from build123d import *

# Parameters (mm, degrees)
SKIZZE1_R                             = 44
AUFSATZ_LINEAR_AUSTRAGEN1_DEPTH       = 4
SCHNITT_LINEAR_START                  = -10
SCHNITT_LINEAR_AUSTRAGEN2_DEPTH       = 10
KREISMUSTER1_COUNT                    = 6
SCHNITT_LINEAR_AUSTRAGEN3_DEPTH       = 4
SCHNITT_LINEAR_AUSTRAGEN3_DEPTH_BACK  = 10
VERRUNDUNG1_R                         = 2
SKIZZE7_R                             = 32
SCHNITT_LINEAR_AUSTRAGEN7_DEPTH       = 0.5
SKIZZE8_R                             = 45
SKIZZE8_R_2                           = 43
AUFSATZ_LINEAR_AUSTRAGEN2_DEPTH       = 6
AUFSATZ_LINEAR_AUSTRAGEN3_DEPTH       = 9
AUFSATZ_LINEAR_AUSTRAGEN3_DEPTH_BACK  = 1
SKIZZE9_R                             = 45
SKIZZE9_R_2                           = 39.5
SKIZZE4_R                             = 21.007106764
AUFSATZ_LINEAR_AUSTRAGEN8_DEPTH       = 6
FASE1_SIZE                            = 3.25
SKIZZE10_R                            = 50
SKIZZE10_R_2                          = 42
SCHNITT_LINEAR_AUSTRAGEN9_DEPTH       = 8
SKIZZE11_R                            = 50
SKIZZE11_R_2                          = 40.9
SCHNITT_LINEAR_AUSTRAGEN10_DEPTH      = 2
SCHNITT_LINEAR_AUSTRAGEN11_DEPTH      = 6
SCHNITT_LINEAR_AUSTRAGEN11_DEPTH_BACK = 6
FASE3_SIZE                            = 2
FASE5_SIZE                            = 2
SKIZZE12_R                            = 2.5
SCHNITT_LINEAR_AUSTRAGEN12_DEPTH      = 79.994520679
VERRUNDUNG2_R                         = 1


with BuildPart() as part:
    # Skizze1 → Aufsatz-Linear austragen1 (new body)
    with BuildSketch(Plane(origin=(0, 0, 0), x_dir=(1, 0, 0), z_dir=(0, 1, 0))):
        with Locations(Location((0, 0, 0), (0, 0, 270))):
            Circle(SKIZZE1_R)
    extrude(amount=AUFSATZ_LINEAR_AUSTRAGEN1_DEPTH)

    # Skizze2 → Schnitt-Linear austragen2 (cut)
    with BuildSketch(Plane(origin=(0, 4, 0), x_dir=(1, 0, 0), z_dir=(0, 1, 0)).offset(SCHNITT_LINEAR_START)):
        with BuildLine():
            ThreePointArc((-30, 0), (-30.647234858, 7.855929826), (-32.571484726, 15.5))
            Line((-32.571484726, 15.5), (-41.179485184, 15.5))
            ThreePointArc((-41.179485184, 15.5), (-44, 0), (-41.179485184, -15.5))
            Line((-41.179485184, -15.5), (-32.571484726, -15.5))
            ThreePointArc((-32.571484726, -15.5), (-30.647234858, -7.855929826), (-30, 0))
        make_face()
    schnitt_linear_austragen2 = extrude(amount=SCHNITT_LINEAR_AUSTRAGEN2_DEPTH, mode=Mode.SUBTRACT)

    # Kreismuster1: Schnitt-Linear austragen2 ×6 about axis
    kreismuster1_axis = Axis((0, 0, 0), (0, 1, 0))
    for i in range(1, KREISMUSTER1_COUNT):
        add(schnitt_linear_austragen2.rotate(kreismuster1_axis, i * 360 / KREISMUSTER1_COUNT), mode=Mode.SUBTRACT)

    # Skizze3 → Schnitt-Linear austragen3 (cut, two sides: drawn at the far end of the back side and taken through both)
    with BuildSketch(Plane.XZ.offset(-SCHNITT_LINEAR_AUSTRAGEN3_DEPTH_BACK)):
        Polygon((15, 8.660254038), (0, 17.320508076), (-15, 8.660254038), (-15, -8.660254038), (0, -17.320508076), (15, -8.660254038), align=None)
    extrude(amount=SCHNITT_LINEAR_AUSTRAGEN3_DEPTH + SCHNITT_LINEAR_AUSTRAGEN3_DEPTH_BACK, mode=Mode.SUBTRACT)

    # Verrundung1
    verrundung1_edges = [part.edges().sort_by_distance(p)[0] for p in [
        (-32.571484726, 2, 15.5),
        (-32.571484726, 2, -15.5),
        (-29.709136122, 2, -20.457733212),
        (-2.862348604, 2, -35.957733212),
        (2.862348604, 2, -35.957733212),
        (29.709136122, 2, -20.457733212),
        (32.571484726, 2, -15.5),
        (32.571484726, 2, 15.5),
        (29.709136122, 2, 20.457733212),
        (2.862348604, 2, 35.957733212),
        (-2.862348604, 2, 35.957733212),
        (-29.709136122, 2, 20.457733212),
    ]]
    fillet(verrundung1_edges, radius=VERRUNDUNG1_R)

    # Skizze7 → Schnitt-Linear austragen7 (cut)
    with BuildSketch(Plane.XZ):
        Circle(SKIZZE7_R)
    extrude(amount=-SCHNITT_LINEAR_AUSTRAGEN7_DEPTH, mode=Mode.SUBTRACT)

    # Skizze8 → Aufsatz-Linear austragen2 (add)
    with BuildSketch(Plane(origin=(0, 4, 0), x_dir=(1, 0, 0), z_dir=(0, 1, 0))):
        with Locations(Location((0, 0, 0), (0, 0, 270))):
            Circle(SKIZZE8_R)
        with Locations(Location((0, 0, 0), (0, 0, 270))):
            Circle(SKIZZE8_R_2, mode=Mode.SUBTRACT)
    extrude(amount=-AUFSATZ_LINEAR_AUSTRAGEN2_DEPTH)



with BuildPart() as body_2:
    # Skizze9 → Aufsatz-Linear austragen3 (new, two sides: drawn at the far end of the back side and taken through both)
    with BuildSketch(Plane.XZ.offset(2).offset(-AUFSATZ_LINEAR_AUSTRAGEN3_DEPTH_BACK)):
        with Locations(Location((0, 0, 0), (0, 0, 90))):
            Circle(SKIZZE9_R)
        with Locations(Location((0, 0, 0), (0, 0, 270))):
            Circle(SKIZZE9_R_2, mode=Mode.SUBTRACT)
    extrude(amount=AUFSATZ_LINEAR_AUSTRAGEN3_DEPTH + AUFSATZ_LINEAR_AUSTRAGEN3_DEPTH_BACK)


with BuildPart() as part_1:
    add(part.part)

    add(body_2.part)  # Aufsatz-Linear austragen8 merges body 2
    # Skizze4 → Aufsatz-Linear austragen8 (add)
    with BuildSketch(Plane(origin=(0, 4, 0), x_dir=(1, 0, 0), z_dir=(0, 1, 0))):
        with Locations(Location((0, 0, 0), (0, 0, 270))):
            Circle(SKIZZE4_R)
    extrude(amount=-AUFSATZ_LINEAR_AUSTRAGEN8_DEPTH)

    # Fase1
    fase1_edges = [part_1.edges().sort_by_distance(p)[0] for p in [
        (0, -1, 39.5),
    ]]
    chamfer(fase1_edges, length=FASE1_SIZE)

    # Skizze10 → Schnitt-Linear austragen9 (cut)
    with BuildSketch(Plane.XZ.offset(11)):
        Circle(SKIZZE10_R)
        with Locations(Location((0, 0, 0), (0, 0, 270))):
            Circle(SKIZZE10_R_2, mode=Mode.SUBTRACT)
    extrude(amount=-SCHNITT_LINEAR_AUSTRAGEN9_DEPTH, mode=Mode.SUBTRACT)

    # Skizze11 → Schnitt-Linear austragen10 (cut)
    with BuildSketch(Plane.XZ.offset(11)):
        with Locations((-1.948563864, 1.772578218)):
            Circle(SKIZZE11_R)
        with Locations(Location((0, 0, 0), (0, 0, 270))):
            Circle(SKIZZE11_R_2, mode=Mode.SUBTRACT)
    extrude(amount=-SCHNITT_LINEAR_AUSTRAGEN10_DEPTH, mode=Mode.SUBTRACT)

    # Skizze3_3 → Schnitt-Linear austragen11 (cut, two sides: drawn at the far end of the back side and taken through both)
    with BuildSketch(Plane.XZ.offset(-SCHNITT_LINEAR_AUSTRAGEN11_DEPTH_BACK)):
        Polygon((15, 8.660254038), (0, 17.320508076), (-15, 8.660254038), (-15, -8.660254038), (0, -17.320508076), (15, -8.660254038), align=None)
    extrude(amount=SCHNITT_LINEAR_AUSTRAGEN11_DEPTH + SCHNITT_LINEAR_AUSTRAGEN11_DEPTH_BACK, mode=Mode.SUBTRACT)

    # Fase3
    fase3_edges = [part_1.edges().sort_by_distance(p)[0] for p in [
        (0, -2, -21.007106764),
    ]]
    chamfer(fase3_edges, length=FASE3_SIZE)

    # Fase5
    fase5_edges = [part_1.edges().sort_by_distance(p)[0] for p in [
        (15, 4, 0),
        (7.5, 4, 12.990381057),
        (-7.5, 4, 12.990381057),
        (-15, 4, 0),
        (-7.5, 4, -12.990381057),
        (7.5, 4, -12.990381057),
    ]]
    chamfer(fase5_edges, length=FASE5_SIZE)

    # Skizze12 → Schnitt-Linear austragen12 (cut, through all)
    with BuildSketch(Plane(origin=(-7.5, 0, 12.990381057), x_dir=(-0.8660254037844387, 0, -0.49999999999999994), z_dir=(0.4999999999999999, 0, -0.8660254037844386))):
        with Locations(Location((0, -4, 0), (0, 0, 354.260829874))):
            Circle(SKIZZE12_R)
    extrude(amount=-SCHNITT_LINEAR_AUSTRAGEN12_DEPTH, mode=Mode.SUBTRACT)

    # Verrundung2
    verrundung2_edges = [part_1.edges().sort_by_distance(p)[0] for p in [
        (40.850402975, -3, 9.759332805),
    ]]
    fillet(verrundung2_edges, radius=VERRUNDUNG2_R)


solid = part_1.part
Design review of the part built by this model. Coordinates are the model's own, in mm. A direction names the side the tool comes from. Give positions to 0.01 mm unless a question says otherwise; leave off trailing zeros.
1. Mouldability with a two-part tool opening along X and no side actions: class faces 5 (the flat face through (23.1, -3, -36.5)), 6 (the flat face through (7.888, 3.014, -13.937)) as +X half, -X half, draft (parallel to the pull), parting line (faces both ways), or undercut.
Solution:
face 5: draft
face 6: undercut
2. Add section A-A, the plane z = 29. State how many separate pieces and enclosed holes the cut face has, then the cut area to 3 significant figures.
Solution:
separate pieces: 3
enclosed holes: 0
area: 166 mm2
3. Tool access review of faces 1 (the flat face through (16, 3, 0)), 2 (the conical face through (-38.715, -4.092, 8.597)), 3 (the flat face through (-8, -2, -13)), 4 (the cylindrical face through (29.49, 2.03, 20.88)): name each direction out of +Z, -Z, +X, -X, +Y, -Y from which nothing blocks a thin tool from reaching the whole face with its end or side.
Solution:
face 1: +Y
face 2: none
face 3: -Y
face 4: +Y, -Y
4. To check wall thickness, follow L1, parallel to X at y = 0.1, z = 0; L2, parallel to Z at x = 0, y = 1.65; L3, parallel to X at y = 1.25, z = -26.5. State the ranges of each line that lie inside material, in increasing order.
Solution:
L1: x = -45 to -43, -21.01 to -15, 15 to 21.01, 43 to 45
L2: z = -45 to -17.32, 17.32 to 45
L3: x = -36.37 to -33.2, -14.12 to 14.12, 33.2 to 36.37
5. For pin 1 Ø19 at (x, z) = (-4, 4.5) entering from -Y; pin 2 Ø2 at (x, y) = (-28, -2) entering from +Z; pin 3 Ø10 at (x, z) = (-25.5, -6) entering from -Y, all flat-tipped, find the tip position at first contact; note any pin that passes through.
Solution:
pin 1: stops at y = -2
pin 2: stops at z = 36
pin 3: stops at y = 0.5
